Check sheet for the modelled part. Datum: model origin and axes. Units: mm. A direction names the side the tool comes from. Coordinates: 2 decimals unless noted, no trailing zeros. Write each loop counter-clockwise with the first axis right and the second up, starting at its lowest first coordinate (ties: lowest second). Pieces come first, ordered by that corner, then holes. Notation, with made-up numbers: (40.25, 52.25) - (66.25, 52.25) arc R26 cw to (66.25, 82.25) - close; hole circle Ø7 at (74.25, 29.5). An arc over 180 degrees is marked (long way). Use one line per item in the form item = value. Start each with the question number.
1. Tool access check on faces 5 (the face through (1, -1, 8.1)), 6 (the face through (10, -1, 6.85)), 7 (the face through (10, -1, 1.25)). Record the directions out of +Z, -Z, +X, -X, +Y, -Y that give a thin tool (end or side, any length) a straight path to the whole face; none if there is none.
2. Cross-section at D-D on z = 6.5. Record the boundary of the cut face in (x, y).
3. Go/stop test with flat-tipped pins: pin 1 Ø0.9 at (x, y) = (4, -0.5) entering from +Z; pin 2 Ø0.6 at (x, y) = (10.5, -1) entering from +Z; pin 3 Ø0.6 at (x, y) = (10.5, -1) entering from -Z. Record where each tip stops, or that it passes through.
4. Cross-section at C-C on x = 9.75. Record the boundary of the cut face in (y, z), then the cut area to 3 significant figures.
5. Draft check along X on faces 1 (the face through (19, -1, 6.2)), 2 (the face through (17, -1, 0.675)), 3 (the face through (14, -1, 7.425)), 4 (the face through (11.99, -0.99, 7.13)). Enter one of: +X half, -X half, draft (parallel to the pull), parting line (faces both ways), or undercut.
6. Cross-section at B-B on z = 0.5. Record the boundary of the cut face in (x, y).
7. Scan lines: line 1 along X through (y, z) = (-1.2, 1); line 2 along Z through (x, y) = (10.25, -0.2); line 3 along Z through (x, y) = (12.5, -0.9) (3 decimals). Record each from-to range of solid material in increasing order.
```python
from build123d import *

# Parameters (mm, degrees)
PAD_DEPTH = 2


with BuildPart() as part:
    # Sketch → Pad (new body)
    with BuildSketch(Plane.XZ):
        Polygon((2, 8.1), (3.6, 7.425), (4.4, 7.425), (5.2, 6.85), (6.8, 6.85), (7.6, 7.425), (8.1, 7.425), (8.4, 6.85), (10, 6.85), (11.6, 6.85), (12.4, 7.425), (13.2, 7.425), (14.8, 7.425), (15.6, 8.1), (16.4, 7.425), (17.2, 7.425), (18, 6.85), (20, 5.55), (20, 4.05), (0, 4.05), (0, 8.1), align=None)
    pad = extrude(amount=PAD_DEPTH)

    # Mirrored: Pad across Sketch Axis8
    add(pad.mirror(Plane(origin=(0, 0, 4.05), x_dir=(0, -1, 0), z_dir=(0, 0, 1))))


solid = part.part
```
Final values:
q1.face_5 = +Z, +X, -X, +Y, -Y
q1.face_6 = +Z, +Y, -Y
q1.face_7 = -Z, +Y, -Y
q2.outline = (0, -2) - (18.54, -2) - (18.54, 0) - (0, 0) - close
q3.pin_1 = 7.45
q3.pin_2 = 6.85
q3.pin_3 = 1.25
q4.outline = (-2, 1.25) - (0, 1.25) - (0, 6.85) - (-2, 6.85) - close
q4.area = 11.2 mm²
q5.face_1 = +X half
q5.face_2 = draft
q5.face_3 = undercut
q5.face_4 = undercut
q6.outline = (0, -2) - (3.19, -2) - (3.19, 0) - (0, 0) - close; (15.01, -2) - (16.19, -2) - (16.19, 0) - (15.01, 0) - close
q7.line_1 = 0 to 4.85, 7.15 to 8.27, 11.95 to 17.65
q7.line_2 = 1.25 to 6.85
q7.line_3 = 0.675 to 7.425
